```python
from build123d import *

# Parameters (mm, degrees)
EXTRUDE_1_DEPTH     = 3
SKETCH_3_R          = 2
CUT_EXTRUDE_1_DEPTH = 3
SKETCH_5_W          = 17.5
SKETCH_5_H          = 8
CUT_EXTRUDE_2_DEPTH = 3
FILLET_1_R          = 1
FILLET_2_R          = 1
CUT_EXTRUDE_3_DEPTH = 10
SKETCH_7_R          = 1.6
CUT_EXTRUDE_4_DEPTH = 10
SKETCH_8_R          = 1.6
CUT_EXTRUDE_5_DEPTH = 10
SKETCH_9_R          = 1.6
CUT_EXTRUDE_6_DEPTH = 3
SKETCH_10_R         = 1.6
CUT_EXTRUDE_7_DEPTH = 3
FILLET_3_R          = 3
FILLET_4_R          = 3
CUT_EXTRUDE_8_DEPTH = 11.6
CUT_EXTRUDE_9_DEPTH = 11.6
FILLET_5_R          = 2


with BuildPart() as part:
    # 草图2 → 凸台-拉伸1 (new body)
    with BuildSketch(Plane.XY):
        with BuildLine():
            Line((-177.154590294, 76.5), (-177.154590294, 66.5))
            ThreePointArc((-177.154590294, 66.5), (-154.308919227, 11.345671067), (-99.154590294, -11.5))
            Line((-99.154590294, -11.5), (-88, -11.5))
            Line((-88, -11.5), (-74.5, -11.5))
            Line((-74.5, -11.5), (-74.5, -3))
            Line((-74.5, -3), (-88, -3))
            Line((-88, -3), (-88, 3))
            Line((-88, 3), (-74.5, 3))
            Line((-74.5, 3), (-74.5, 21.5))
            Line((-74.5, 21.5), (-77.5, 21.5))
            Line((-77.5, 21.5), (-77.5, 29.5))
            Line((-77.5, 29.5), (-74.5, 29.5))
            Line((-74.5, 29.5), (-74.5, 50))
            Line((-74.5, 50), (-99.154590294, 50))
            Line((-99.154590294, 50), (-99.154590294, 76.5))
            Line((-99.154590294, 76.5), (-177.154590294, 76.5))
        make_face()
    extrude(amount=EXTRUDE_1_DEPTH)

    # 草图3 → 切除-拉伸1 (cut)
    with BuildSketch(Plane.XY.offset(3)):
        with Locations((-86, 3)):
            Circle(SKETCH_3_R)
        with Locations((-86, -3)):
            Circle(SKETCH_3_R)
    extrude(amount=-CUT_EXTRUDE_1_DEPTH, mode=Mode.SUBTRACT)

    # 草图5 → 切除-拉伸2 (cut)
    with BuildSketch(Plane.XY.offset(3)):
        with Locations((-168.404590294, 72.5)):
            Rectangle(SKETCH_5_W, SKETCH_5_H)
    extrude(amount=-CUT_EXTRUDE_2_DEPTH, mode=Mode.SUBTRACT)

    # 圆角1
    fillet_1_edges = [part.edges().sort_by_distance(p)[0] for p in [
        (-159.654590294, 68.5, 1.5),
    ]]
    fillet(fillet_1_edges, radius=FILLET_1_R)

    # 圆角2
    fillet_2_edges = [part.edges().sort_by_distance(p)[0] for p in [
        (-74.5, 29.5, 1.5),
        (-77.5, 29.5, 1.5),
        (-77.5, 21.5, 1.5),
        (-74.5, 21.5, 1.5),
    ]]
    fillet(fillet_2_edges, radius=FILLET_2_R)

    # 草图6 → 切除-拉伸3 (cut)
    with BuildSketch(Plane.XY.offset(3)):
        Polygon((-174.154590294, 69.502681713), (-174.154590294, 33.470652635), (-188.349025992, 74.64093898), align=None)
    extrude(amount=-CUT_EXTRUDE_3_DEPTH, mode=Mode.SUBTRACT)

    # 草图7 → 切除-拉伸4 (cut)
    with BuildSketch(Plane.XY.offset(3)):
        with Locations((-122, 6)):
            Circle(SKETCH_7_R)
        with Locations((-142, 6)):
            Circle(SKETCH_7_R)
    extrude(amount=-CUT_EXTRUDE_4_DEPTH, mode=Mode.SUBTRACT)

    # 草图8 → 切除-拉伸5 (cut)
    with BuildSketch(Plane.XY.offset(3)):
        with Locations((-170.287955794, 46.10283567)):
            Circle(SKETCH_8_R)
        with Locations((-159.021847878, 23.00389133)):
            Circle(SKETCH_8_R)
        with Locations((-93.154590294, -7.5)):
            Circle(SKETCH_8_R)
        with Locations((-114.540055415, -5.882922454)):
            Circle(SKETCH_8_R)
    extrude(amount=-CUT_EXTRUDE_5_DEPTH, mode=Mode.SUBTRACT)

    # 草图9 → 切除-拉伸6 (cut)
    with BuildSketch(Plane.XY.offset(3)):
        with Locations((-103.154590294, 72.5)):
            Circle(SKETCH_9_R)
        with Locations((-111.154590294, 72.5)):
            Circle(SKETCH_9_R)
        with Locations((-111.154590294, 64.5)):
            Circle(SKETCH_9_R)
        with Locations((-103.154590294, 64.5)):
            Circle(SKETCH_9_R)
    extrude(amount=-CUT_EXTRUDE_6_DEPTH, mode=Mode.SUBTRACT)

    # 草图10 → 切除-拉伸7 (cut)
    with BuildSketch(Plane.XY.offset(3)):
        with Locations((-122.010091835, 57)):
            Circle(SKETCH_10_R)
        with Locations((-154.010091835, 57)):
            Circle(SKETCH_10_R)
    extrude(amount=-CUT_EXTRUDE_7_DEPTH, mode=Mode.SUBTRACT)

    # 圆角3
    fillet_3_edges = [part.edges().sort_by_distance(p)[0] for p in [
        (-99.154590294, 50, 1.5),
    ]]
    fillet(fillet_3_edges, radius=FILLET_3_R)

    # 圆角4
    fillet_4_edges = [part.edges().sort_by_distance(p)[0] for p in [
        (-174.154590294, 68.5, 1.5),
        (-174.154590294, 45.075714714, 1.5),
        (-99.154590294, 76.5, 1.5),
        (-74.5, 50, 1.5),
        (-74.5, 3, 1.5),
        (-74.5, -3, 1.5),
        (-74.5, -11.5, 1.5),
        (-159.654590294, 76.5, 1.5),
    ]]
    fillet(fillet_4_edges, radius=FILLET_4_R)

    # 草图13 → 切除-拉伸8 (cut)
    with BuildSketch(Plane.XY.offset(3)):
        with BuildLine():
            Line((-166.665700491, 48), (-141.270501777, 48))
            ThreePointArc((-141.270501777, 48), (-139.774924791, 44.913234948), (-138.053500491, 41.946491381))
            Line((-138.053500491, 41.946491381), (-157.497103519, 27.819886884))
            ThreePointArc((-157.497103519, 27.819886884), (-162.885217731, 37.544739224), (-166.665700491, 48))
        make_face()
        with BuildLine():
            ThreePointArc((-134.526788978, 37.092389415), (-131.483826087, 33.776606028), (-128.131412478, 30.774046183))
            Line((-128.131412478, 30.774046183), (-142.021368274, 11.160688967))
            ThreePointArc((-142.021368274, 11.160688967), (-148.351253457, 16.703530912), (-153.970392005, 22.965784918))
            Line((-153.970392005, 22.965784918), (-134.526788978, 37.092389415))
        make_face()
        with BuildLine():
            Line((-127.680893946, 48), (-111.060471194, 48))
            ThreePointArc((-111.060471194, 48), (-105.946714568, 45.574727054), (-100.383436414, 44.53434642))
            Line((-100.383436414, 44.53434642), (-99.407755019, 32.500942548))
            ThreePointArc((-99.407755019, 32.500942548), (-115.498385615, 36.685903426), (-127.680893946, 48))
        make_face()
        with BuildLine():
            Line((-133.154590294, 72.5), (-133.154590294, 66.5))
            ThreePointArc((-133.154590294, 66.5), (-133.042454912, 63.740900214), (-132.706788434, 61))
            Line((-132.706788434, 61), (-121.498246805, 61))
            Line((-121.498246805, 61), (-115.154590294, 65.382793706))
            Line((-115.154590294, 65.382793706), (-115.154590294, 72.5))
            Line((-115.154590294, 72.5), (-133.154590294, 72.5))
        make_face()
        with BuildLine():
            ThreePointArc((-123.234931322, 27.306414096), (-117.609516434, 24.364317958), (-111.632610014, 22.224735756))
            Line((-111.632610014, 22.224735756), (-114.443614375, 9))
            Line((-114.443614375, 9), (-136.199324912, 9))
            Line((-136.199324912, 9), (-123.234931322, 27.306414096))
        make_face()
        with BuildLine():
            ThreePointArc((-105.763724409, 20.977265611), (-102.467762347, 20.619471549), (-99.154590294, 20.5))
            Line((-99.154590294, 20.5), (-98.434705623, 20.5))
            Line((-98.434705623, 20.5), (-96.488759677, -3.5))
            Line((-96.488759677, -3.5), (-99.154590294, -3.5))
            ThreePointArc((-99.154590294, -3.5), (-104.977776216, -3.257368827), (-110.760593955, -2.531157306))
            Line((-110.760593955, -2.531157306), (-105.763724409, 20.977265611))
        make_face()
    extrude(amount=-CUT_EXTRUDE_8_DEPTH, mode=Mode.SUBTRACT)

    # 草图14 → 切除-拉伸9 (cut)
    with BuildSketch(Plane.XY.offset(3)):
        with BuildLine():
            Line((-145.154590294, 72.5), (-145.154590294, 66.5))
            ThreePointArc((-145.154590294, 66.5), (-145.072019197, 63.745054808), (-144.824602337, 61))
            Line((-144.824602337, 61), (-169.154590294, 61))
            Line((-169.154590294, 61), (-145.154590294, 72.5))
        make_face()
        Polygon((-94.482583074, 46), (-93.387988479, 32.5), (-81.154590294, 32.5), (-78.5, 35.154590294), (-78.5, 46), align=None)
        Polygon((-92.415015506, 20.5), (-81.154590294, 20.5), (-78.5, 17.845409706), (-78.5, 7), (-91.320420912, 7), align=None)
    extrude(amount=-CUT_EXTRUDE_9_DEPTH, mode=Mode.SUBTRACT)

    # 圆角5
    fillet_5_edges = [part.edges().sort_by_distance(p)[0] for p in [
        (-111.632610014, 22.224735756, 1.5),
        (-114.443614375, 9, 1.5),
        (-136.199324912, 9, 1.5),
        (-123.234931322, 27.306414096, 1.5),
        (-115.154590294, 72.5, 1.5),
        (-115.154590294, 65.382793706, 1.5),
        (-121.498246805, 61, 1.5),
        (-132.706788434, 61, 1.5),
        (-133.154590294, 72.5, 1.5),
        (-128.131412478, 30.774046183, 1.5),
        (-142.021368274, 11.160688967, 1.5),
        (-153.970392005, 22.965784918, 1.5),
        (-134.526788978, 37.092389415, 1.5),
        (-138.053500491, 41.946491381, 1.5),
        (-157.497103519, 27.819886884, 1.5),
        (-166.665700491, 48, 1.5),
        (-98.434705623, 20.5, 1.5),
        (-96.488759677, -3.5, 1.5),
        (-110.760593955, -2.531157306, 1.5),
        (-105.763724409, 20.977265611, 1.5),
        (-111.060471194, 48, 1.5),
        (-100.383436414, 44.53434642, 1.5),
        (-99.407755019, 32.500942548, 1.5),
        (-127.680893946, 48, 1.5),
        (-81.154590294, 20.5, 1.5),
        (-78.5, 17.845409706, 1.5),
        (-78.5, 7, 1.5),
        (-91.320420912, 7, 1.5),
        (-92.415015506, 20.5, 1.5),
        (-78.5, 35.154590294, 1.5),
        (-81.154590294, 32.5, 1.5),
        (-93.387988479, 32.5, 1.5),
        (-94.482583074, 46, 1.5),
        (-78.5, 46, 1.5),
        (-144.824602337, 61, 1.5),
        (-169.154590294, 61, 1.5),
        (-145.154590294, 72.5, 1.5),
        (-141.270501777, 48, 1.5),
    ]]
    fillet(fillet_5_edges, radius=FILLET_5_R)


solid = part.part
```
Work out the finished part from the listing and answer in its coordinate system (mm). A direction names the side the tool comes from. Coordinates: 2 decimals unless noted, no trailing zeros. Loops run counter-clockwise (first coordinate to the right, second up) from the corner with the lowest first, then second, coordinate; pieces in that order, holes last.
1) For a pull along Y with two mould halves and no side action, classify faces 4 (the flat face through (-86, 46, 2)), 5 (the flat face through (-129, 76.5, 1)), 6 (the flat face through (-74.5, 13, 1)) as +Y half, -Y half, draft (parallel to the pull), parting line (faces both ways), or undercut.
Results:
face 4: undercut
face 5: +Y half
face 6: draft
2) Section A-A (y = 57) is taken. Give the vertices of the cut face in (x, z).
Results:
outline: (-174.15, 0) - (-155.61, 0) - (-155.61, 3) - (-174.15, 3) - close; (-152.41, 0) - (-123.61, 0) - (-123.61, 3) - (-152.41, 3) - close; (-120.41, 0) - (-99.15, 0) - (-99.15, 3) - (-120.41, 3) - close
3) For faces 1 (the flat face through (-159.655, 71, 2)), 2 (the flat face through (-78.5, 40, 2)), 3 (the flat face through (-87, 50, 1)), determine the directions among +Z, -Z, +X, -X, +Y, -Y from which every point of the face is accessible in a straight line to the end or side of a thin tool.
Results:
face 1: +Z, -Z, -X, +Y
face 2: +Z, -Z
face 3: +Z, -Z, +X, +Y
4) Consider probe 1 along Y at (x, z) = (-83, 1.1); probe 2 along X at (y, z) = (64.5, 1.4); probe 3 along Y at (x, z) = (-144, 1.9). Determine where each line is inside the solid, lowest interval first.
Results:
probe 1: y = -11.5 to -3, 3 to 7, 20.5 to 32.5, 46 to 50
probe 2: x = -174.15 to -161.68, -145.11 to -133.1, -116.43 to -112.75, -109.55 to -104.75, -101.55 to -99.15
probe 3: y = 2.68 to 12.75, 30.21 to 37.63, 48 to 76.5
5) Section B-B (z = 2.15) is taken. Give the number of separate pieces and of enclosed holes in the cut face, plus the area to 3 significant figures.
Results:
separate pieces: 1
enclosed holes: 21
area: 4,520 mm2
6) Flat-ended cylindrical pins translate along their axes: pin 1 (1.5 mm diameter, centred on y = 68.5, z = 2, fed in from -X); pin 2 (1.5 mm diameter, centred on y = 40, z = 2, fed in from -X); pin 3 (1.5 mm diameter, centred on x = -163.5, z = 1, fed in from +Y); pin 4 (5 mm diameter, centred on x = -122.01, y = 57, fed in from -Z). Find the tip coordinate at first contact, or state that the pin passes through.
Results:
pin 1: stops at x = -173.14
pin 2: stops at x = -172.78
pin 3: stops at y = 68.5
pin 4: stops at z = 0
